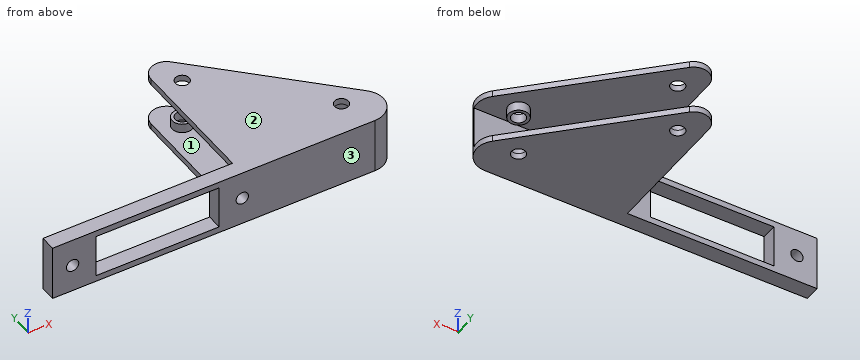
```python
from build123d import *

# Parameters (mm, degrees)
SKETCH1_W           = 116.445688755
SKETCH1_H           = 18
SKETCH1_R           = 2
SKETCH1_W_2         = 40
SKETCH1_H_2         = 14
BOSS_EXTRUDE1_DEPTH = 5
SKETCH2_R           = 2.25
BOSS_EXTRUDE2_DEPTH = 2
BOSS_EXTRUDE3_START = -2
SKETCH4_R           = 2.25
BOSS_EXTRUDE3_DEPTH = 2
FILLET2_R           = 7
FILLET3_R           = 5
SKETCH6_R           = 3.25
SKETCH6_R_2         = 2.25
BOSS_EXTRUDE4_DEPTH = 3
BOSS_EXTRUDE5_START = 3
SKETCH7_R           = 3.25
SKETCH7_R_2         = 2.25
BOSS_EXTRUDE5_DEPTH = 3


with BuildPart() as part:
    # Sketch1 → Boss-Extrude1 (new body)
    with BuildSketch(Plane(origin=(0, 0, 0), x_dir=(1, 0, 0), z_dir=(0, 1, 0))):
        with Locations((22.222844378, 0)):
            Rectangle(SKETCH1_W, SKETCH1_H)
        with Locations(Location((-29.5, 0, 0), (0, 0, 270))):
            Circle(SKETCH1_R, mode=Mode.SUBTRACT)
        with Locations(Location((25.5, 0, 0), (0, 0, 270))):
            Circle(SKETCH1_R, mode=Mode.SUBTRACT)
        with Locations((-2, 0)):
            Rectangle(SKETCH1_W_2, SKETCH1_H_2, mode=Mode.SUBTRACT)
    extrude(amount=BOSS_EXTRUDE1_DEPTH)

    # Sketch2 → Boss-Extrude2 (add)
    # profile 1 of 2: a face of its own
    with BuildSketch(Plane.XY.offset(9)):
        Polygon((85.482180719, 0), (80.445688755, 5), (80.445688755, 0), align=None)
    # profile 2 of 2: a face of its own
    with BuildSketch(Plane.XY.offset(9)):
        Polygon((25.445687742, 59.601497833), (25.445688755, 5), (80.445688755, 5), align=None)
        with Locations((64.445688755, 11)):
            Circle(SKETCH2_R, mode=Mode.SUBTRACT)
        with Locations((32.447088786, 42.64)):
            Circle(SKETCH2_R, mode=Mode.SUBTRACT)
    extrude(amount=-BOSS_EXTRUDE2_DEPTH)

    # Sketch4 → Boss-Extrude3 (add)
    # profile 1 of 2: a face of its own
    with BuildSketch(Plane(origin=(0, 0, -9), x_dir=(-1, 0, 0), z_dir=(0, 0, -1)).offset(BOSS_EXTRUDE3_START)):
        Polygon((-25.445687742, 59.601497833), (-80.445688755, 5), (-25.445687742, 5), align=None)
        with Locations(Location((-64.445688755, 11, 0), (0, 0, 180))):
            Circle(SKETCH4_R, mode=Mode.SUBTRACT)
        with Locations(Location((-32.447088786, 42.64, 0), (0, 0, 180))):
            Circle(SKETCH4_R, mode=Mode.SUBTRACT)
    # profile 2 of 2: a face of its own
    with BuildSketch(Plane(origin=(0, 0, -9), x_dir=(-1, 0, 0), z_dir=(0, 0, -1)).offset(BOSS_EXTRUDE3_START)):
        Polygon((-80.445688755, 5), (-85.482180719, 0), (-80.445688755, 0), align=None)
    extrude(amount=BOSS_EXTRUDE3_DEPTH)

    # Fillet2
    # the kernel refuses this fillet: 7 mm, written as the material it takes off along each edge
    with BuildSketch(Plane(origin=(85.482180719, 0, 35.466936405), x_dir=(-1, 0, 0), z_dir=(0, 0, -1))) as fillet2_piece_1:
        with BuildLine():
            CenterArc((FILLET2_R * 2.42668208026, FILLET2_R), FILLET2_R, 134.791677578, 135.208322422)
            Line((FILLET2_R * 1.72215094548, FILLET2_R * 1.70967307975), (0, 0))
            Line((0, 0), (FILLET2_R * 2.42668208026, 0))
        make_face()
    extrude(amount=86.933872809, mode=Mode.SUBTRACT)

    # Fillet3
    fillet3_edges = [part.edges().sort_by_distance(p)[0] for p in [
        (25.445687742, 59.601497833, 8),
        (25.445687742, 59.601497833, -8),
    ]]
    fillet(fillet3_edges, radius=FILLET3_R)

    # Sketch6 → Boss-Extrude4 (add)
    with BuildSketch(Plane(origin=(0, 0, 7), x_dir=(-1, 0, 0), z_dir=(0, 0, -1))):
        with Locations(Location((-64.445688755, 11, 0), (0, 0, 180))):
            Circle(SKETCH6_R)
        with Locations(Location((-64.445688755, 11, 0), (0, 0, 180))):
            Circle(SKETCH6_R_2, mode=Mode.SUBTRACT)
    extrude(amount=BOSS_EXTRUDE4_DEPTH)

    # Sketch7 → Boss-Extrude5 (add)
    # profile 1 of 2: a face of its own
    with BuildSketch(Plane.XY.offset(-7).offset(BOSS_EXTRUDE5_START)):
        with Locations(Location((32.447088786, 42.64, 0), (0, 0, 180))):
            Circle(SKETCH7_R)
        with Locations((32.447088786, 42.64)):
            Circle(SKETCH7_R_2, mode=Mode.SUBTRACT)
    # profile 2 of 2: a face of its own
    with BuildSketch(Plane.XY.offset(-7).offset(BOSS_EXTRUDE5_START)):
        with Locations((64.445688755, 11)):
            Circle(SKETCH7_R)
        with Locations((64.445688755, 11)):
            Circle(SKETCH7_R_2, mode=Mode.SUBTRACT)
    extrude(amount=-BOSS_EXTRUDE5_DEPTH)


solid = part.part
```
Check sheet for the modelled part. Datum: model origin and axes. Units: mm. Face numbers are marked on the shaded views. Coordinates: 2 decimals unless noted, no trailing zeros. Order: outer loops, then holes, each group sorted by start corner. A loop starts at its lowest first (then second) coordinate and runs counter-clockwise, first axis right, second up. Notation, with made-up numbers: M -3,34 L 49,34 A27 cw 49,66 Z; hole C 50,56.5 d8. An arc over 180 degrees is marked long. One line per question, with ' | ' between items. Start each with the question number.
Item 1: Gauge pin test, flat ends, axial feed: P1, Ø1.6, axis at y = 18.5, z = 8, coming from the -X side; P2, Ø5.5, axis at x = 35.5, z = 3.5, coming from the +Y side. Record the tip position at first contact, or that the pin passes through.
Item 2: Sectioned sample at D-D on y = 42.64. Record the cut outline in (x, z).
Item 3: Material ranges on line 1 (Z direction, x = 45, y = 30); line 2 (Y direction, x = 19, z = 5.25); line 3 (X direction, y = 11, z = 4.85), recorded low to high.
Item 4: Sectioned sample at A-A on x = -0.5. Record the cut outline in (y, z), and give its area (3 significant figures).
Item 5: Sectioned sample at C-C on y = 26. Record the cut outline in (x, z), and give its area (3 significant figures).
Item 6: Mould release check, pull along Y, two halves, no side actions. Record for the marked faces 1, 2 and 3: pulls with the +Y half, pulls with the -Y half, needs draft (parallel to the pull), parting line crosses it, or undercut.
Item 7: Sectioned sample at B-B on z = 0. Record the cut outline in (x, y).
Answer below:
1) P1: stops at x = 25.45 | P2: stops at y = 5
2) outline: M 25.45,-9 L 30.2,-9 L 30.2,-4 L 29.2,-4 L 29.2,-7 L 25.45,-7 Z; M 25.45,7 L 30.2,7 L 30.2,9 L 25.45,9 Z; M 34.7,-9 L 42.53,-9 L 42.53,-7 L 35.7,-7 L 35.7,-4 L 34.7,-4 Z; M 34.7,7 L 42.53,7 L 42.53,9 L 34.7,9 Z
3) line 1: z = -9 to -7, 7 to 9 | line 2: y = 0 to 5 | line 3: x = 61.2 to 62.2, 66.7 to 67.7
4) outline: M 0,-9 L 5,-9 L 5,-7 L 0,-7 Z; M 0,7 L 5,7 L 5,9 L 0,9 Z | area: 20.0 mm^2
5) outline: M 25.45,-9 L 59.29,-9 L 59.29,-7 L 25.45,-7 Z; M 25.45,7 L 59.29,7 L 59.29,9 L 25.45,9 Z | area: 135 mm^2
6) face 1: undercut | face 2: needs draft | face 3: pulls with the -Y half
7) outline: M -36,0 L -31.5,0 L -31.5,5 L -36,5 Z; M -27.5,0 L -22,0 L -22,5 L -27.5,5 Z; M 18,0 L 23.5,0 L 23.5,5 L 18,5 Z; M 27.5,0 L 68.5,0 A7 ccw 75.2,5 L 27.5,5 Z
